Verification items for the finished model (mm, model axes). A direction names the side the tool comes from. Coordinates: 2 decimals unless noted, no trailing zeros. Order: outer loops, then holes, each group sorted by start corner. A loop starts at its lowest first (then second) coordinate and runs counter-clockwise, first axis right, second up. Notation, with made-up numbers: M 65,-28 L 122,-28 A11 cw 122,-22 Z; hole C 41,15 d4. An arc over 180 degrees is marked long. Return JSON: item names as keys, results as strings. Group by question number.
1. Set-up check for faces 1 (the flat face through (-13.9, -2.984, 78.916)), 2 (the flat face through (11, 2, 12)): record each of +Z, -Z, +X, -X, +Y, -Y from which the full face is reachable in a straight line by a thin tool's end or side.
2. Material ranges on line 1 along X through (y, z) = (-35, 43); line 2 along Z through (x, y) = (12, -2); line 3 along Z through (x, y) = (-12.5, -18.5), recorded low to high.
3. Section check C-C, the plane x = 21. Record the cut outline in (y, z).
4. Mould release check, pull along Z, two halves, no side actions. Record for faces 3 (the cylindrical face through (13.41, -6.75, 78.92)), 4 (the flat face through (2.6, -14.5, 85)), 5 (the flat face through (6, -4.072, 16)): +Z half, -Z half, draft (parallel to the pull), parting line (faces both ways), or undercut.
5. Section check A-A, the plane z = 43. Record the cut outline in (x, y), plus the area to 3 significant figures.
6. Gauge pin test, flat ends, axial feed: pin 1 (6 mm diameter, centred on x = 14.5, z = 27.5, fed in from +Y); pin 2 (11 mm diameter, centred on x = 9.65, y = -12.66, fed in from +Z). Record the tip position at first contact, or that the pin passes through.
7. Section check B-B, the plane y = 3. Record the cut outline in (x, z).
8. Section check D-D, the plane y = -29. Record the cut outline in (x, z).
```python
from build123d import *

# Parameters (mm, degrees)
SKETCH_1_R          = 7
EXTRUDE_1_DEPTH     = 85
CUT_EXTRUDE_1_DEPTH = 107.24319241
SKETCH_3_R          = 8
CUT_EXTRUDE_2_DEPTH = 96.804760434


with BuildPart() as part:
    # 스케치1 → 보스-돌출1 (new body)
    with BuildSketch(Plane.XY):
        Polygon((-23.351828972, -14), (-4.179415178, 8.344827586), (27.820584822, 8.344827586), (27.820584822, -38), (-23.351828972, -38), align=None)
        with Locations((9.648171028, -12.655172414)):
            Circle(SKETCH_1_R, mode=Mode.SUBTRACT)
    extrude(amount=EXTRUDE_1_DEPTH)

    # 스케치2 → 컷-돌출1 (cut, through all)
    with BuildSketch(Plane.ZY.offset(23.351828972)):
        Polygon((12, 8.344827586), (12, -4.071985155), (20, -4.071985155), (20, -26), (73, -26), (73, 8.344827586), align=None)
    extrude(amount=-CUT_EXTRUDE_1_DEPTH, mode=Mode.SUBTRACT)

    # 스케치3 → 컷-돌출2 (cut, through all)
    with BuildSketch(Plane(origin=(0, -26, 0), x_dir=(1, 0, 0), z_dir=(0, 1, 0))):
        with Locations(Location((-1.179415178, -43, 0), (0, 0, 270))):
            Circle(SKETCH_3_R)
    extrude(amount=-CUT_EXTRUDE_2_DEPTH, mode=Mode.SUBTRACT)


solid = part.part
```
Answers follow:
{
 "1": {"face 1": "+Z, -Z, -X, +Y", "face 2": "+X, -X, +Y"},
 "2": {"line 1": "-23.35 to -9.18, 6.82 to 27.82", "line 2": "0 to 12, 73 to 85", "line 3": "0 to 20, 73 to 85"},
 "3": {"outline": "M -38,0 L 8.34,0 L 8.34,12 L -4.07,12 L -4.07,20 L -26,20 L -26,73 L 8.34,73 L 8.34,85 L -38,85 Z"},
 "4": {"face 3": "draft", "face 4": "+Z half", "face 5": "undercut"},
 "5": {"outline": "M -23.35,-38 L -9.18,-38 L -9.18,-26 L -23.35,-26 Z; M 6.82,-38 L 27.82,-38 L 27.82,-26 L 6.82,-26 Z", "area": "422 mm^2"},
 "6": {"pin 1": "y = -26", "pin 2": "through"},
 "7": {"outline": "M -8.77,0 L 27.82,0 L 27.82,12 L -8.77,12 Z; M -8.77,73 L 27.82,73 L 27.82,85 L -8.77,85 Z"},
 "8": {"outline": "M -23.35,0 L 27.82,0 L 27.82,85 L -23.35,85 Z; hole C -1.18,43 d16"}
}
